```python
from build123d import *

# Parameters (mm, degrees)
SKETCH_1_W             = 42.3
SKETCH_1_H             = 42.3
EXTRUDE_1_DEPTH        = 48
SKETCH_2_R             = 11
EXTRUDE_2_DEPTH        = 2
SKETCH_3_R             = 2.5
EXTRUDE_3_DEPTH        = 22
CHAMFER_1_SIZE         = 5
HOLE_WIZARD_M3_1_D     = 2.5
HOLE_WIZARD_M3_1_DEPTH = 6
HOLE_WIZARD_M3_1_TIP   = 0.751075774
SKETCH_7_OUTSIDE_W     = 63.022
SKETCH_7_OUTSIDE_H     = 63.022
SKETCH_7_OUTSIDE_W_2   = 38
SKETCH_7_OUTSIDE_H_2   = 38
CUT_EXTRUDE_2_DEPTH    = 25
SKETCH_8_W             = 6.700255884
SKETCH_8_H             = 1.991967966
CUT_EXTRUDE_3_DEPTH    = 20


with BuildPart() as part:
    # 草图1 → 凸台-拉伸1 (new body)
    with BuildSketch(Plane.XY):
        with Locations((21.15, -21.15)):
            Rectangle(SKETCH_1_W, SKETCH_1_H)
    extrude(amount=EXTRUDE_1_DEPTH)

    # 草图2 → 凸台-拉伸2 (add)
    with BuildSketch(Plane.XY.offset(48)):
        with Locations((21.15, -21.15)):
            Circle(SKETCH_2_R)
    extrude(amount=EXTRUDE_2_DEPTH)

    # 草图3 → 凸台-拉伸3 (add)
    with BuildSketch(Plane.XY.offset(50)):
        with Locations((21.15, -21.15)):
            Circle(SKETCH_3_R)
    extrude(amount=EXTRUDE_3_DEPTH)

    # 倒角1
    chamfer_1_edges = [part.edges().sort_by_distance(p)[0] for p in [
        (0, 0, 24),
        (42.3, 0, 24),
        (42.3, -42.3, 24),
        (0, -42.3, 24),
    ]]
    chamfer(chamfer_1_edges, length=CHAMFER_1_SIZE)

    # M3 螺纹孔1
    with Locations(Plane(origin=(5.65, -5.65, 48), x_dir=(1, 0, 0), z_dir=(0, 0, 1))):
        with Locations((0, 0), (0, -31), (31, -31), (31, 0)):
            Hole(HOLE_WIZARD_M3_1_D / 2, depth=HOLE_WIZARD_M3_1_DEPTH)
            with Locations((0, 0, -(HOLE_WIZARD_M3_1_DEPTH + HOLE_WIZARD_M3_1_TIP / 2))):  # 118° drill point
                Cone(0, HOLE_WIZARD_M3_1_D / 2, HOLE_WIZARD_M3_1_TIP, mode=Mode.SUBTRACT)

    # 草图7 outside → 切除-拉伸2 (cut)
    with BuildSketch(Plane(origin=(0, 0, 10), x_dir=(-1, 0, 0), z_dir=(0, 0, -1))):
        with Locations((-21.15, -21.15)):
            Rectangle(SKETCH_7_OUTSIDE_W, SKETCH_7_OUTSIDE_H)
        with Locations((-21.15, -21.15)):
            Rectangle(SKETCH_7_OUTSIDE_W_2, SKETCH_7_OUTSIDE_H_2, mode=Mode.SUBTRACT)
    extrude(amount=-CUT_EXTRUDE_2_DEPTH, mode=Mode.SUBTRACT)

    # 草图8 → 切除-拉伸3 (cut)
    with BuildSketch(Plane.XY.offset(72)):
        with Locations((21.681661742, -18.154016017)):
            Rectangle(SKETCH_8_W, SKETCH_8_H)
    extrude(amount=-CUT_EXTRUDE_3_DEPTH, mode=Mode.SUBTRACT)


solid = part.part
```
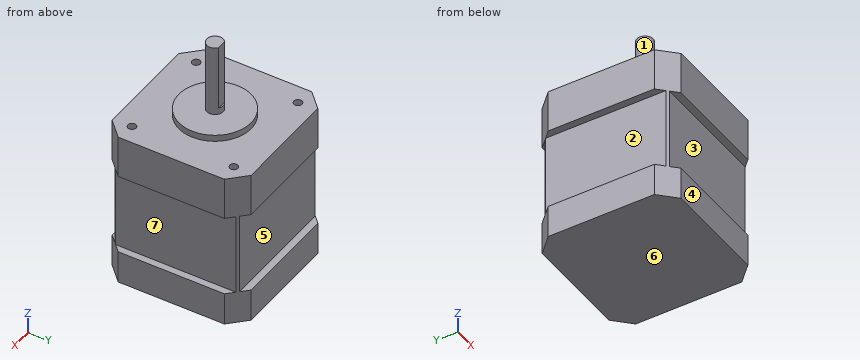
Input: part model. Units: mm. Frame: model coordinates. Face numbers are marked on the shaded views. A direction names the side the tool comes from. Round coordinates to 2 decimals unless told otherwise and drop trailing zeros. Write each loop counter-clockwise with the first axis right and the second up, starting at its lowest first coordinate (ties: lowest second). Pieces come first, ordered by that corner, then holes. Notation, with made-up numbers: (12.5, 43) - (49.5, 43) arc R12 cw to (49.5, 66) - close; hole circle Ø11 at (85, 21.5). An arc over 180 degrees is marked (long way). Write item = value, one per line.
(1) Pull-direction query (Z, two-part tool) for the marked faces 4, 5, 6 and 7; classes: +Z half, -Z half, draft (parallel to the pull), parting line (faces both ways), or undercut.
Geometry check:
face_4 = draft
face_5 = undercut
face_6 = -Z half
face_7 = undercut
(2) Section query A-A on z = 47. Output: boundary loops of the cut face in (x, y).
Geometry check:
outline = (0, -37.3) - (5, -42.3) - (37.3, -42.3) - (42.3, -37.3) - (42.3, -5) - (37.3, 0) - (5, 0) - (0, -5) - close; hole circle Ø2.5 at (5.65, -36.65); hole circle Ø2.5 at (5.65, -5.65); hole circle Ø2.5 at (36.65, -36.65); hole circle Ø2.5 at (36.65, -5.65)
(3) Contact query for flat-ended pins moving along their axis: pin 1 Ø1.5 at (x, z) = (15.5, 13) entering from +Y; pin 2 Ø1 at (y, z) = (-5, 30.5) entering from -X; pin 3 Ø7.5 at (x, z) = (19, 16.5) entering from -Y. Output: stop coordinate, or through.
Geometry check:
pin_1 = -2.15
pin_2 = 2.15
pin_3 = -40.15
(4) Section query C-C on x = 21.15. Output: boundary loops of the cut face in (y, z), then the cut area to 3 significant figures.
Geometry check:
outline = (-42.3, 0) - (0, 0) - (0, 10) - (-2.15, 10) - (-2.15, 35) - (0, 35) - (0, 48) - (-10.15, 48) - (-10.15, 50) - (-18.65, 50) - (-18.65, 52) - (-19.15, 52) - (-19.15, 72) - (-23.65, 72) - (-23.65, 50) - (-32.15, 50) - (-32.15, 48) - (-42.3, 48) - (-42.3, 35) - (-40.15, 35) - (-40.15, 10) - (-42.3, 10) - close
area = 2,070 mm^2
(5) Section query B-B on y = -21.15. Output: boundary loops of the cut face in (x, z), then the cut area to 3 significant figures.
Geometry check:
outline = (0, 0) - (42.3, 0) - (42.3, 10) - (40.15, 10) - (40.15, 35) - (42.3, 35) - (42.3, 48) - (32.15, 48) - (32.15, 50) - (23.65, 50) - (23.65, 72) - (18.65, 72) - (18.65, 50) - (10.15, 50) - (10.15, 48) - (0, 48) - (0, 35) - (2.15, 35) - (2.15, 10) - (0, 10) - close
area = 2,080 mm^2
(6) Access query for the marked faces 1, 2 and 3. Directions: +Z, -Z, +X, -X, +Y, -Y. A direction counts if a zero-diameter tool reaches every point of the face in a straight line with its end or side. Return the directions, or none.
Geometry check:
face_1 = +Z
face_2 = -X, +Y, -Y
face_3 = +X, -X, -Y
(7) Section query D-D on z = 20.5. Output: boundary loops of the cut face in (x, y).
Geometry check:
outline = (2.15, -39.45) - (2.85, -40.15) - (39.45, -40.15) - (40.15, -39.45) - (40.15, -2.85) - (39.45, -2.15) - (2.85, -2.15) - (2.15, -2.85) - close
(8) Material intervals for probe 1 along Y at (x, z) = (36.65, 44.75); probe 2 along X at (y, z) = (-5.65, 46.1); probe 3 along Y at (x, z) = (36, 46), sorted ascending.
Geometry check:
probe_1 = -42.3 to -37.9, -35.4 to -6.9, -4.4 to 0
probe_2 = 0 to 4.4, 6.9 to 35.4, 37.9 to 42.3
probe_3 = -42.3 to -37.72, -35.58 to -6.72, -4.58 to 0
